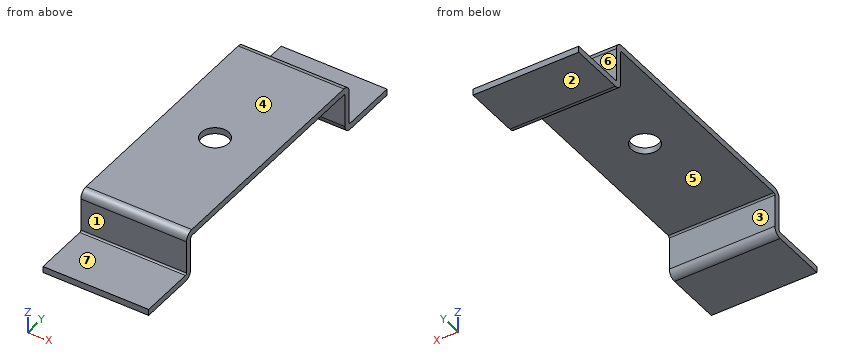
```python
from build123d import *

# Parameters (mm, degrees)
SKETCH_1_W                         = 50
SKETCH_1_H                         = 110
SM_BASE_FLANGE_1_DEPTH             = 3
SM_EDGE_FLANGE_1_STRIP_W           = 13.4732
SM_EDGE_FLANGE_1_STRIP_H           = 3
SM_EDGE_FLANGE_1_STRIP_CUT_DEPTH   = 50
SM_EDGE_FLANGE_1_STRIP_2_W         = 13.4732
SM_EDGE_FLANGE_1_STRIP_2_H         = 3
SM_EDGE_FLANGE_1_STRIP_CUT_2_DEPTH = 50
SM_EDGE_FLANGE_1_DEPTH             = 50
SM_EDGE_FLANGE_1_BEND_DEPTH        = 50
SM_EDGE_FLANGE_2_STRIP_W           = 13.4732
SM_EDGE_FLANGE_2_STRIP_H           = 3
SM_EDGE_FLANGE_2_STRIP_CUT_DEPTH   = 50
SM_EDGE_FLANGE_2_STRIP_2_W         = 13.4732
SM_EDGE_FLANGE_2_STRIP_2_H         = 3
SM_EDGE_FLANGE_2_STRIP_CUT_2_DEPTH = 50
SM_EDGE_FLANGE_2_DEPTH             = 50
SM_EDGE_FLANGE_2_BEND_DEPTH        = 50
SKETCH_18_R                        = 6.5
CUT_EXTRUDE_1_DEPTH                = 151.429385427


# Sheet-metal steps are written as plain solids
with BuildPart() as part:
    # Sketch 1 → 基体-法兰1 (new body)
    with BuildSketch(Plane.XY):
        with Locations((25, 55)):
            Rectangle(SKETCH_1_W, SKETCH_1_H)
    extrude(amount=-SM_BASE_FLANGE_1_DEPTH)

    # 边线-法兰1 strip (across the edge) → 边线-法兰1 strip cut (cut)
    with BuildSketch(Plane(origin=(0, 110, -3), x_dir=(0, -1, 0), z_dir=(1, 0, 0))):
        with Locations((-6, -1.5)):
            Rectangle(SM_EDGE_FLANGE_1_STRIP_W, SM_EDGE_FLANGE_1_STRIP_H)
    extrude(amount=SM_EDGE_FLANGE_1_STRIP_CUT_DEPTH, mode=Mode.SUBTRACT)

    # 边线-法兰1 strip 2 (across the edge) → 边线-法兰1 strip cut 2 (cut)
    with BuildSketch(Plane(origin=(50, 0, -3), x_dir=(0, 1, 0), z_dir=(-1, 0, 0))):
        with Locations((-6, -1.5)):
            Rectangle(SM_EDGE_FLANGE_1_STRIP_2_W, SM_EDGE_FLANGE_1_STRIP_2_H)
    extrude(amount=SM_EDGE_FLANGE_1_STRIP_CUT_2_DEPTH, mode=Mode.SUBTRACT)

    # 边线-法兰1 section (across the edge) → 边线-法兰1 (add)
    with BuildSketch(Plane(origin=(0, 110, -3), x_dir=(0, -1, 0), z_dir=(1, 0, 0))):
        with BuildLine():
            Line((-3, 0.7366), (-3, 17))
            Line((-3, 17), (0, 17))
            Line((0, 17), (0, 0.7366))
            ThreePointArc((0, 0.7366), (0.215745145, 0.215745145), (0.7366, 0))
            Line((0.7366, 0), (0.7366, -3))
            ThreePointArc((0.7366, -3), (-1.905575199, -1.905575199), (-3, 0.7366))
        make_face()
    extrude(amount=SM_EDGE_FLANGE_1_DEPTH)

    # 边线-法兰1 section 2 (across the edge) → 边线-法兰1 bend (add)
    with BuildSketch(Plane(origin=(50, 0, -3), x_dir=(0, 1, 0), z_dir=(-1, 0, 0))):
        with BuildLine():
            Line((-3, 0.7366), (-3, 17))
            Line((-3, 17), (0, 17))
            Line((0, 17), (0, 0.7366))
            ThreePointArc((0, 0.7366), (0.215745145, 0.215745145), (0.7366, 0))
            Line((0.7366, 0), (0.7366, -3))
            ThreePointArc((0.7366, -3), (-1.905575199, -1.905575199), (-3, 0.7366))
        make_face()
    extrude(amount=SM_EDGE_FLANGE_1_BEND_DEPTH)

    # 边线-法兰2 strip (across the edge) → 边线-法兰2 strip cut (cut)
    with BuildSketch(Plane(origin=(0, -3, -20), x_dir=(0, 0, 1), z_dir=(1, 0, 0))):
        with Locations((-6, -1.5)):
            Rectangle(SM_EDGE_FLANGE_2_STRIP_W, SM_EDGE_FLANGE_2_STRIP_H)
    extrude(amount=SM_EDGE_FLANGE_2_STRIP_CUT_DEPTH, mode=Mode.SUBTRACT)

    # 边线-法兰2 strip 2 (across the edge) → 边线-法兰2 strip cut 2 (cut)
    with BuildSketch(Plane(origin=(50, 113, -20), x_dir=(0, 0, 1), z_dir=(-1, 0, 0))):
        with Locations((-6, -1.5)):
            Rectangle(SM_EDGE_FLANGE_2_STRIP_2_W, SM_EDGE_FLANGE_2_STRIP_2_H)
    extrude(amount=SM_EDGE_FLANGE_2_STRIP_CUT_2_DEPTH, mode=Mode.SUBTRACT)

    # 边线-法兰2 section (across the edge) → 边线-法兰2 (add)
    with BuildSketch(Plane(origin=(0, -3, -20), x_dir=(0, 0, 1), z_dir=(1, 0, 0))):
        with BuildLine():
            Line((-3, 0.7366), (-3, 27))
            Line((-3, 27), (0, 27))
            Line((0, 27), (0, 0.7366))
            ThreePointArc((0, 0.7366), (0.215745145, 0.215745145), (0.7366, 0))
            Line((0.7366, 0), (0.7366, -3))
            ThreePointArc((0.7366, -3), (-1.905575199, -1.905575199), (-3, 0.7366))
        make_face()
    extrude(amount=SM_EDGE_FLANGE_2_DEPTH)

    # 边线-法兰2 section 2 (across the edge) → 边线-法兰2 bend (add)
    with BuildSketch(Plane(origin=(50, 113, -20), x_dir=(0, 0, 1), z_dir=(-1, 0, 0))):
        with BuildLine():
            Line((-3, 0.7366), (-3, 27))
            Line((-3, 27), (0, 27))
            Line((0, 27), (0, 0.7366))
            ThreePointArc((0, 0.7366), (0.215745145, 0.215745145), (0.7366, 0))
            Line((0.7366, 0), (0.7366, -3))
            ThreePointArc((0.7366, -3), (-1.905575199, -1.905575199), (-3, 0.7366))
        make_face()
    extrude(amount=SM_EDGE_FLANGE_2_BEND_DEPTH)

    # 草图18 → 切除-拉伸1 (cut, through all)
    with BuildSketch(Plane.XY):
        with Locations((25, 55)):
            Circle(SKETCH_18_R)
    extrude(amount=-CUT_EXTRUDE_1_DEPTH, mode=Mode.SUBTRACT)


solid = part.part
```
The model under review builds one solid part; all positions refer to its coordinate system, in mm. Face numbers are marked on the shaded views. A direction names the side the tool comes from. Round coordinates to 2 decimals unless told otherwise and drop trailing zeros. Order: outer loops, then holes, each group sorted by start corner. A loop starts at its lowest first (then second) coordinate and runs counter-clockwise, first axis right, second up.
Item 1: Add section A-A, the plane y = 55. State the section outline as (x, z) points, and give its area (3 significant figures).
Working result:
outline: (0, -3) - (18.5, -3) - (18.5, 0) - (0, 0) - close; (31.5, -3) - (50, -3) - (50, 0) - (31.5, 0) - close
area: 111 mm2
Item 2: Draft analysis for pull direction Y (two halves, no side actions). For the marked faces 1, 2 and 3, state which applies: released by +Y, released by -Y, zero draft, split by the parting line, or undercut.
Working result:
face 1: released by -Y
face 2: zero draft
face 3: undercut
Item 3: To check wall thickness, follow probe 1 along Y at (x, z) = (43.5, -12.75); probe 2 along Z at (x, y) = (25, 13); probe 3 along Y at (x, z) = (25, -1.75). State the ranges of each line that lie inside material, in increasing order.
Working result:
probe 1: y = -3 to 0, 110 to 113
probe 2: z = -3 to 0
probe 3: y = -2.43 to 48.5, 61.5 to 112.43
Item 4: Machinability: for the marked faces 4, 5, 6 and 7, which of the approach directions +Z, -Z, +X, -X, +Y, -Y give a long, thin tool a straight path to every point of the face, cutting with its end or side? Answer none if there is none.
Working result:
face 4: +Z, +X, -X, +Y, -Y
face 5: -Z, +X, -X
face 6: +Z, +X, -X, +Y
face 7: +Z, +X, -X, -Y
Item 5: Add section D-D, the plane x = 47. State the section outline as (y, z) points, and give its area (3 significant figures).
Working result:
outline: (-30, -23) - (-3.74, -23) arc R3.74 ccw to (0, -19.26) - (0, -3.74) arc R0.74 cw to (0.74, -3) - (109.26, -3) arc R0.74 cw to (110, -3.74) - (110, -19.26) arc R3.74 ccw to (113.74, -23) - (140, -23) - (140, -20) - (113.74, -20) arc R0.74 cw to (113, -19.26) - (113, -3.74) arc R3.74 ccw to (109.26, 0) - (0.74, 0) arc R3.74 ccw to (-3, -3.74) - (-3, -19.26) arc R0.74 cw to (-3.74, -20) - (-30, -20) - close
area: 618 mm2
Item 6: Add section C-C, the plane z = -11.75. State the section outline as (x, y) points, and give its area (3 significant figures).
Working result:
outline: (0, -3) - (50, -3) - (50, 0) - (0, 0) - close; (0, 110) - (50, 110) - (50, 113) - (0, 113) - close
area: 300 mm2
Item 7: For pin 1 (10 mm diameter, centred on x = 37, z = -10, fed in from +Y); pin 2 (4 mm diameter, centred on x = 21, z = -5.5, fed in from -Y); pin 3 (3 mm diameter, centred on x = 31, y = 3, fed in from +Z), all flat-tipped, find the tip position at first contact; note any pin that passes through.
Working result:
pin 1: stops at y = 113
pin 2: stops at y = -3
pin 3: stops at z = 0
Item 8: Add section B-B, the plane x = 25. State the section outline as (y, z) points, and give its area (3 significant figures).
Working result:
outline: (-30, -23) - (-3.74, -23) arc R3.74 ccw to (0, -19.26) - (0, -3.74) arc R0.74 cw to (0.74, -3) - (48.5, -3) - (48.5, 0) - (0.74, 0) arc R3.74 ccw to (-3, -3.74) - (-3, -19.26) arc R0.74 cw to (-3.74, -20) - (-30, -20) - close; (61.5, -3) - (109.26, -3) arc R0.74 cw to (110, -3.74) - (110, -19.26) arc R3.74 ccw to (113.74, -23) - (140, -23) - (140, -20) - (113.74, -20) arc R0.74 cw to (113, -19.26) - (113, -3.74) arc R3.74 ccw to (109.26, 0) - (61.5, 0) - close
area: 579 mm2
